CAD build for the part. Positions are in the model's coordinates, mm. A direction names the side the tool comes from. Give positions to 0.01 mm unless a question says otherwise; leave off trailing zeros. Loops run counter-clockwise (first coordinate to the right, second up) from the corner with the lowest first, then second, coordinate; pieces in that order, holes last. Notation, with made-up numbers: (75, 23.25) - (102, 23.25) arc R10 cw to (102, 39.25) - close; hole circle Ø9 at (30.25, -30.75). An arc over 180 degrees is marked (long way). Return JSON: item names as keys, results as strings.
from build123d import *

# Parameters (mm, degrees)
SKETCH1_W          = 31.75
SKETCH1_H          = 50.8
SKETCH1_W_2        = 3.175
SKETCH1_H_2        = 3.175
CUT_EXTRUDE1_DEPTH = 83.672025196


with BuildPart() as part:
    # Sketch1 → Revolve1 (revolve)
    with BuildSketch(Plane.XY, mode=Mode.PRIVATE) as revolve1_sk:
        with Locations((0, 25.4)):
            Rectangle(SKETCH1_W, SKETCH1_H)
        with Locations((-14.2875, 52.3875)):
            Rectangle(SKETCH1_W_2, SKETCH1_H_2)
        with Locations((14.2875, 52.3875)):
            Rectangle(SKETCH1_W_2, SKETCH1_H_2)
    revolve(revolve1_sk.sketch.rotate(Axis((-15.875, 0, 0), (1, 0, 0)), 180), axis=Axis((-15.875, 0, 0), (1, 0, 0)))

    # Sketch2 → Cut-Extrude1 (cut, through all)
    with BuildSketch(Plane.ZY.offset(15.875)):
        with BuildLine():
            Line((-6.745565901, 8.004027254), (-5.556686402, 5.668081023))
            ThreePointArc((-5.556686402, 5.668081023), (3.600316682, -7.074010605), (-1.312280039, 7.828271032))
            Line((-1.312280039, 7.828271032), (-2.632559092, 10.422395062))
            Line((-2.632559092, 10.422395062), (-6.745565901, 8.004027254))
        make_face()
    extrude(amount=-CUT_EXTRUDE1_DEPTH, mode=Mode.SUBTRACT)


solid = part.part
1. Cut at A-A, the plane y = 0. Write the cut outline in (x, z) (1 decimal).
Values follow:
{"outline": "(-15.9, -54) - (-12.7, -54) - (-12.7, -50.8) - (12.7, -50.8) - (12.7, -54) - (15.9, -54) - (15.9, -7.9) - (-15.9, -7.9) - close; (-15.9, 7.9) - (15.9, 7.9) - (15.9, 54) - (12.7, 54) - (12.7, 50.8) - (-12.7, 50.8) - (-12.7, 54) - (-15.9, 54) - close"}
2. Cut at D-D, the plane z = -46.5. Write the cut outline in (x, y) (3 decimals), plus the area to 3 significant figures.
Values follow:
{"outline": "(-15.875, -27.405) - (-12.7, -27.405) - (-12.7, -20.455) - (12.7, -20.455) - (12.7, -27.405) - (15.875, -27.405) - (15.875, 27.405) - (12.7, 27.405) - (12.7, 20.455) - (-12.7, 20.455) - (-12.7, 27.405) - (-15.875, 27.405) - close", "area": "1,390 mm²"}
3. Drop flat-ended pins along their axis: P1, Ø10, axis at x = -3.5, z = 39, coming from the +Y side; P2, Ø8, axis at x = 7, y = -16, coming from the -Z side; P3, Ø9.5, axis at y = 0, z = 0, coming from the +X side; P4, Ø8, axis at x = -2.5, y = -7.5, coming from the +Z side. Give the stop position or say it passes through.
Values follow:
{"P1": "stops at y = 37.74", "P2": "stops at z = -49.36", "P3": "passes through", "P4": "stops at z = 50.68"}
4. Cut at C-C, the plane x = 9.5. Write the cut outline in (y, z) (1 decimal).
Values follow:
{"outline": "circle Ø101.6 at (0, 0); hole (5.7, -5.6) - (8, -6.7) - (10.4, -2.6) - (7.8, -1.3) arc R7.9 ccw (long way) to start"}
5. Which spindle directions (+Z, -Z, +X, -X, +Y, -Y) get a long thin tool onto all of the face, cutting with end or side? Do faces 1 (the face through (-0.22, 9.23, -4.66)), 2 (the face through (0.18, -23.44, 45.07)), 3 (the face through (15.875, 11, -1)). Say none if no direction does.
Values follow:
{"face 1": "+X, -X", "face 2": "none", "face 3": "+Z, -Z, +X, +Y, -Y"}
6. Pull direction Z, two halves, no side cores. Call faces 4 (the face through (-0.222, 9.107, -1.963)), 5 (the face through (-14.27, 39.78, -36.48)), 6 (the face through (-12.7, 32, 40)): +Z half, -Z half, draft (parallel to the pull), parting line (faces both ways), or undercut.
Values follow:
{"face 4": "undercut", "face 5": "parting line", "face 6": "draft"}
7. Drill centre lines: probe 1 along Z at (x, y) = (0.5, 0); probe 2 along X at (y, z) = (-35.5, -38.5) (3 decimals); probe 3 along Z at (x, y) = (13, 0.5). Where is each one in solid material? Low to high.
Values follow:
{"probe 1": "z = -50.8 to -7.94, 7.94 to 50.8", "probe 2": "x = -15.875 to -12.7, 12.7 to 15.875", "probe 3": "z = -53.97 to -7.92, 7.92 to 53.97"}
